from build123d import *

# Parameters (mm, degrees)
SKETCH1_R           = 1.5
BOSS_EXTRUDE1_DEPTH = 10
BOSS_EXTRUDE2_DEPTH = 10


with BuildPart() as part:
    # Sketch1 → Boss-Extrude1 (new body)
    with BuildSketch(Plane.XY):
        with BuildLine():
            Line((31.5, -15), (-31.5, -15))
            Line((-31.5, -15), (-31.5, -29.533829211))
            ThreePointArc((-31.5, -29.533829211), (-31.792893219, -30.240935993), (-32.5, -30.533829211))
            Line((-32.5, -30.533829211), (-40.5, -30.533829211))
            ThreePointArc((-40.5, -30.533829211), (-41.207106781, -30.240935993), (-41.5, -29.533829211))
            Line((-41.5, -29.533829211), (-41.5, -15.067658423))
            ThreePointArc((-41.5, -15.067658423), (-56.533829211, -0.033829211), (-41.5, 15))
            Line((-41.5, 15), (-41.5, 29.466170789))
            ThreePointArc((-41.5, 29.466170789), (-41.207106781, 30.17327757), (-40.5, 30.466170789))
            Line((-40.5, 30.466170789), (-32.5, 30.466170789))
            ThreePointArc((-32.5, 30.466170789), (-31.792893219, 30.17327757), (-31.5, 29.466170789))
            Line((-31.5, 29.466170789), (-31.5, 15))
            Line((-31.5, 15), (31.5, 15))
            Line((31.5, 15), (31.5, 29.466170789))
            ThreePointArc((31.5, 29.466170789), (31.792893219, 30.17327757), (32.5, 30.466170789))
            Line((32.5, 30.466170789), (40.5, 30.466170789))
            ThreePointArc((40.5, 30.466170789), (41.207106781, 30.17327757), (41.5, 29.466170789))
            Line((41.5, 29.466170789), (41.5, 15))
            ThreePointArc((41.5, 15), (56.533829211, -0.033829211), (41.5, -15.067658423))
            Line((41.5, -15.067658423), (41.5, -29.533829211))
            ThreePointArc((41.5, -29.533829211), (41.207106781, -30.240935993), (40.5, -30.533829211))
            Line((40.5, -30.533829211), (32.5, -30.533829211))
            ThreePointArc((32.5, -30.533829211), (31.792893219, -30.240935993), (31.5, -29.533829211))
            Line((31.5, -29.533829211), (31.5, -15))
        make_face()
        with Locations((-49, -0.033829211)):
            Circle(SKETCH1_R, mode=Mode.SUBTRACT)
        with Locations(Location((49, -0.033829211, 0), (0, 0, 180))):
            Circle(SKETCH1_R, mode=Mode.SUBTRACT)
    extrude(amount=BOSS_EXTRUDE1_DEPTH)

    # Sketch2 → Boss-Extrude2 (add)
    with BuildSketch(Plane.XY.offset(10)):
        with BuildLine():
            Line((-33.499984323, -25.533829211), (-39.499984323, -25.533829211))
            ThreePointArc((-39.499984323, -25.533829211), (-40.207091104, -25.240935993), (-40.499984323, -24.533829211))
            Line((-40.499984323, -24.533829211), (-40.499984323, 24.466170789))
            ThreePointArc((-40.499984323, 24.466170789), (-40.207091104, 25.17327757), (-39.499984323, 25.466170789))
            Line((-39.499984323, 25.466170789), (-33.499984323, 25.466170789))
            ThreePointArc((-33.499984323, 25.466170789), (-32.792877542, 25.17327757), (-32.499984323, 24.466170789))
            Line((-32.499984323, 24.466170789), (-32.499984323, -24.533829211))
            ThreePointArc((-32.499984323, -24.533829211), (-32.792877542, -25.240935993), (-33.499984323, -25.533829211))
        make_face()
        with BuildLine():
            Line((33.499984323, 25.466170789), (39.499984323, 25.466170789))
            ThreePointArc((39.499984323, 25.466170789), (40.207091104, 25.17327757), (40.499984323, 24.466170789))
            Line((40.499984323, 24.466170789), (40.499984323, -24.533829211))
            ThreePointArc((40.499984323, -24.533829211), (40.207091104, -25.240935993), (39.499984323, -25.533829211))
            Line((39.499984323, -25.533829211), (33.499984323, -25.533829211))
            ThreePointArc((33.499984323, -25.533829211), (32.792877542, -25.240935993), (32.499984323, -24.533829211))
            Line((32.499984323, -24.533829211), (32.499984323, 24.466170789))
            ThreePointArc((32.499984323, 24.466170789), (32.792877542, 25.17327757), (33.499984323, 25.466170789))
        make_face()
    extrude(amount=BOSS_EXTRUDE2_DEPTH)


solid = part.part
For this review, take the finished solid that the model builds, in its own axes (mm). A direction names the side the tool comes from. Round coordinates to 2 decimals unless told otherwise and drop trailing zeros. Order: outer loops, then holes, each group sorted by start corner. A loop starts at its lowest first (then second) coordinate and runs counter-clockwise, first axis right, second up. Notation, with made-up numbers: (69.25, 64.5) -> (115.25, 64.5) arc R28 cw to (115.25, 97.5) -> close; hole circle Ø2 at (5, 70.25). An arc over 180 degrees is marked (long way). Write item = value, one per line. Start each with the question number.
1) To check wall thickness, follow line 1 (X direction, y = 20.5, z = 5); line 2 (X direction, y = -7.5, z = 12.25); line 3 (Z direction, x = -47.5, y = -13). State the ranges of each line that lie inside material, in increasing order. Write a range as from..to.
2) Take a section at A-A on z = 17.25. State the section outline as (x, y) points, plus the area to 3 significant figures.
3) Take a section at D-D on x = 35.5. State the section outline as (y, z) points.
4) Tool access review of faces 4 (the face through (40.5, 0, 15)), 5 (the face through (-41.5, -22, 5)), 6 (the face through (0, -15, 5)), 7 (the face through (-32.5, 0, 15)), 8 (the face through (41.5, -22, 5)): name each direction out of +Z, -Z, +X, -X, +Y, -Y from which nothing blocks a thin tool from reaching the whole face with its end or side.
5) The part is to be moulded in two halves that separate along Y. For faces 1 (the face through (37, -30.534, 5)), 2 (the face through (50.5, -0.1, 4.9)), 3 (the face through (-31.5, 22, 5)), say which applies: +Y half, -Y half, draft (parallel to the pull), parting line (faces both ways), or undercut.
6) Take a section at C-C on z = 8.25. State the section outline as (x, y) points.
7) Take a section at B-B on x = -49. State the section outline as (y, z) points.
8) Insertion check: pin 1 (11 mm diameter, centred on y = -9, z = 16, fed in from +X); pin 2 (2 mm diameter, centred on y = 14, z = 6, fed in from -X); pin 3 (5 mm diameter, centred on y = 3.5, z = 15.5, fed in from -X). Each pin has a flat end and moves straight along its axis. Give the tip position at first contact, or say it passes through.
Verdict:
q1.line_1 = -41.5..-31.5, 31.5..41.5
q1.line_2 = -40.5..-32.5, 32.5..40.5
q1.line_3 = 0..10
q2.outline = (-40.5, -24.53) arc R1 ccw to (-39.5, -25.53) -> (-33.5, -25.53) arc R1 ccw to (-32.5, -24.53) -> (-32.5, 24.47) arc R1 ccw to (-33.5, 25.47) -> (-39.5, 25.47) arc R1 ccw to (-40.5, 24.47) -> close; (32.5, -24.53) arc R1 ccw to (33.5, -25.53) -> (39.5, -25.53) arc R1 ccw to (40.5, -24.53) -> (40.5, 24.47) arc R1 ccw to (39.5, 25.47) -> (33.5, 25.47) arc R1 ccw to (32.5, 24.47) -> close
q2.area = 814 mm2
q3.outline = (-30.53, 0) -> (30.47, 0) -> (30.47, 10) -> (25.47, 10) -> (25.47, 20) -> (-25.53, 20) -> (-25.53, 10) -> (-30.53, 10) -> close
q4.face_4 = +Z, +X, +Y, -Y
q4.face_5 = +Z, -Z, -X, -Y
q4.face_6 = +Z, -Z, -Y
q4.face_7 = +Z, +Y, -Y
q4.face_8 = +Z, -Z, +X, -Y
q5.face_1 = -Y half
q5.face_2 = undercut
q5.face_3 = draft
q6.outline = (-41.5, -29.53) arc R1 ccw to (-40.5, -30.53) -> (-32.5, -30.53) arc R1 ccw to (-31.5, -29.53) -> (-31.5, -15) -> (31.5, -15) -> (31.5, -29.53) arc R1 ccw to (32.5, -30.53) -> (40.5, -30.53) arc R1 ccw to (41.5, -29.53) -> (41.5, -15.07) arc R15.03 ccw to (41.5, 15) -> (41.5, 29.47) arc R1 ccw to (40.5, 30.47) -> (32.5, 30.47) arc R1 ccw to (31.5, 29.47) -> (31.5, 15) -> (-31.5, 15) -> (-31.5, 29.47) arc R1 ccw to (-32.5, 30.47) -> (-40.5, 30.47) arc R1 ccw to (-41.5, 29.47) -> (-41.5, 15) arc R15.03 ccw to (-41.5, -15.07) -> close; hole circle Ø3 at (-49, -0.03); hole circle Ø3 at (49, -0.03)
q7.outline = (-13.06, 0) -> (-1.53, 0) -> (-1.53, 10) -> (-13.06, 10) -> close; (1.47, 0) -> (13, 0) -> (13, 10) -> (1.47, 10) -> close
q8.pin_1 = 40.5
q8.pin_2 = -48.99
q8.pin_3 = -40.5
